Verification items for this drawing (mm, ordinates from the low corner). A direction names the side the tool comes from. Coordinates: 2 decimals unless noted, no trailing zeros. Write each loop counter-clockwise with the first axis right and the second up, starting at its lowest first coordinate (ties: lowest second). Pieces come first, ordered by that corner, then holes.
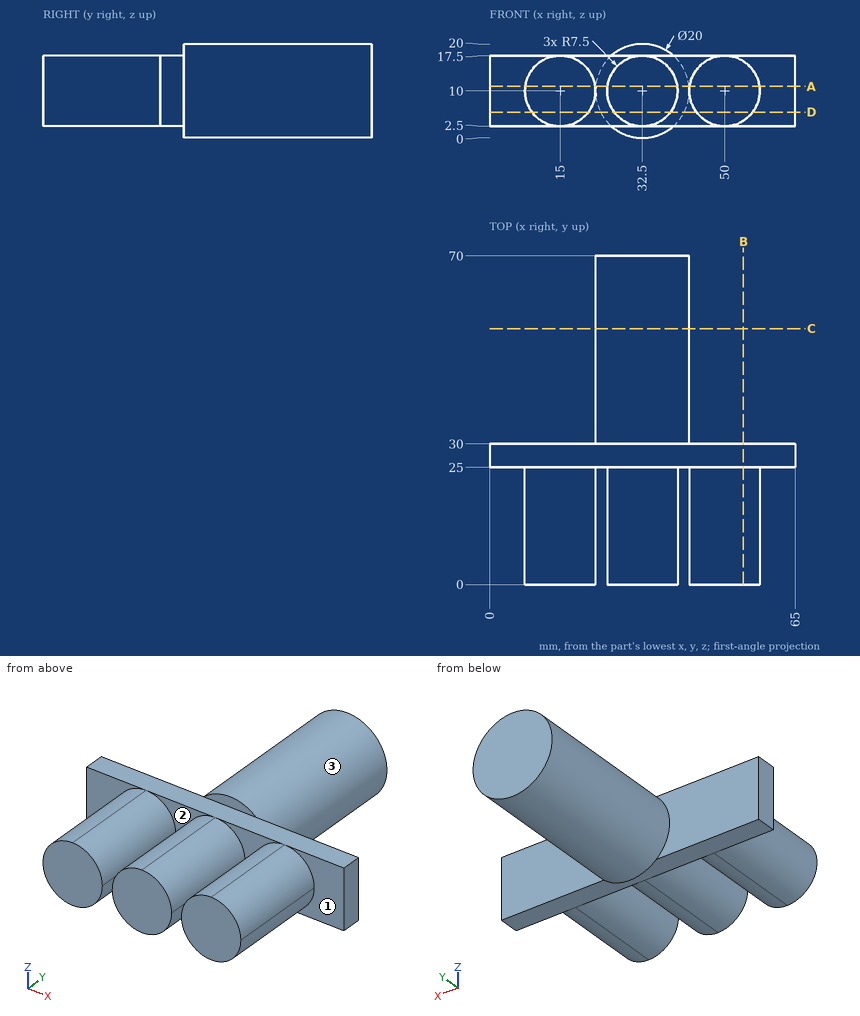
1. Thickness scan on line 1 along X through (y, z) = (6.5, 15.5); line 2 along X through (y, z) = (3, 4.25); line 3 along Y through (x, z) = (40, 16.5). Record the ranges inside material, lowest first.
Computed values:
line 1: x = 9.9 to 20.1, 27.4 to 37.6, 44.9 to 55.1
line 2: x = 10.18 to 19.82, 27.68 to 37.32, 45.18 to 54.82
line 3: y = 25 to 70
2. Sectioned sample at A-A, the plane z = 11. Record the boundary of the cut face in (x, y), and give its area (3 significant figures).
Computed values:
outline: (0, 25) - (7.57, 25) - (7.57, 0) - (22.43, 0) - (22.43, 25) - (25.07, 25) - (25.07, 0) - (39.93, 0) - (39.93, 25) - (42.57, 25) - (42.57, 0) - (57.43, 0) - (57.43, 25) - (65, 25) - (65, 30) - (42.45, 30) - (42.45, 70) - (22.55, 70) - (22.55, 30) - (0, 30) - close
area: 2,240 mm2
3. Sectioned sample at D-D, the plane z = 5.5. Record the boundary of the cut face in (x, y), and give its area (3 significant figures).
Computed values:
outline: (0, 25) - (9, 25) - (9, 0) - (21, 0) - (21, 25) - (26.5, 25) - (26.5, 0) - (38.5, 0) - (38.5, 25) - (44, 25) - (44, 0) - (56, 0) - (56, 25) - (65, 25) - (65, 30) - (41.43, 30) - (41.43, 70) - (23.57, 70) - (23.57, 30) - (0, 30) - close
area: 1,940 mm2
4. Sectioned sample at C-C, the plane y = 54.5. Record the boundary of the cut face in (x, z), and give its area (3 significant figures).
Computed values:
outline: circle Ø20 at (32.5, 10)
area: 314 mm2
5. Access from +Z, -Z, +X, -X, +Y, -Y to the whole of each face (thin tool, end or side, straight path). Record for the marked faces 1, 2 and 3.
Computed values:
face 1: +X, -Y
face 2: -Y
face 3: +Y
6. Sectioned sample at B-B, the plane x = 54. Record the boundary of the cut face in (y, z), and give its area (3 significant figures).
Computed values:
outline: (0, 3.66) - (25, 3.66) - (25, 2.5) - (30, 2.5) - (30, 17.5) - (25, 17.5) - (25, 16.34) - (0, 16.34) - close
area: 392 mm2
7. Gauge pin test, flat ends, axial feed: pin 1 Ø1 at (y, z) = (32.5, 6.5) entering from -X; pin 2 Ø12 at (x, z) = (53, 12.5) entering from +Y; pin 3 Ø4 at (x, y) = (21, 27.5) entering from -Z. Record the tip position at first contact, or that the pin passes through.
Computed values:
pin 1: stops at x = 22.96
pin 2: stops at y = 30
pin 3: stops at z = 2.5
